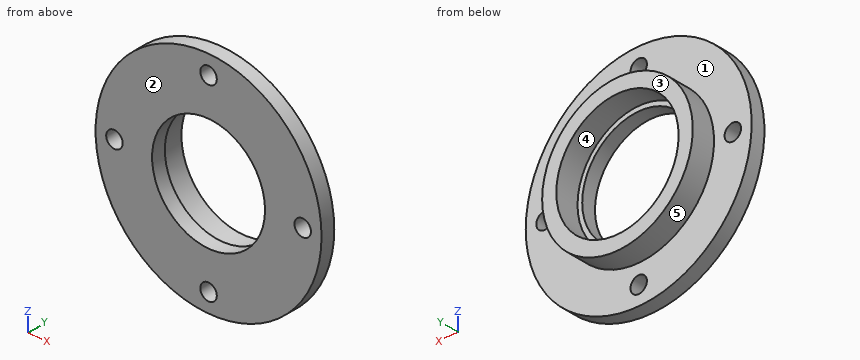
```python
from build123d import *

# Parameters (mm, degrees)
CUT_EXTRUDE_1_DEPTH      = 35.307433597
CUT_EXTRUDE_1_DEPTH_BACK = 35.307433597
SKETCH_2_R               = 1.75


with BuildPart() as part:
    # 草图1 → 旋转1 (revolve)
    with BuildSketch(Plane.XY, mode=Mode.PRIVATE) as revolve_1_sk:
        Polygon((-12, 0), (-24, 0), (-24, 3), (-16, 3), (-16, 8), (-13, 8), (-13, 3), (-12, 3), align=None)
    revolve(revolve_1_sk.sketch.rotate(Axis((0, -271.309816207, 0), (0, 1, 0)), 180), axis=Axis((0, -271.309816207, 0), (0, 1, 0)))

    # 草图2 → 切除-拉伸1 (cut, two sides: drawn at the far end of the back side and taken through both)
    with BuildSketch(Plane(origin=(0, 3, 0), x_dir=(1, 0, 0), z_dir=(0, 1, 0)).offset(-CUT_EXTRUDE_1_DEPTH_BACK)):
        with Locations(Location((0, 20, 0), (0, 0, 180))):
            Circle(SKETCH_2_R)
        with Locations(Location((20, 0, 0), (0, 0, 180))):
            Circle(SKETCH_2_R)
        with Locations(Location((0, -20, 0), (0, 0, 180))):
            Circle(SKETCH_2_R)
        with Locations(Location((-20, 0, 0), (0, 0, 180))):
            Circle(SKETCH_2_R)
    extrude(amount=CUT_EXTRUDE_1_DEPTH + CUT_EXTRUDE_1_DEPTH_BACK, mode=Mode.SUBTRACT)


solid = part.part
```
Geometry check sheet. Reference: the model listing, model coordinates, mm. Face numbers are marked on the shaded views. A direction names the side the tool comes from. Round coordinates to 2 decimals unless told otherwise and drop trailing zeros. Loops run counter-clockwise (first coordinate to the right, second up) from the corner with the lowest first, then second, coordinate; pieces in that order, holes last. Notation, with made-up numbers: M -11,48.25 L 24,48.25 A20 ccw 24,55.25 Z; hole C 3,37.25 d4. An arc over 180 degrees is marked long. Return JSON: item names as keys, results as strings. Group by question number.
(1) Set-up check for the marked faces 1 and 2: record each of +Z, -Z, +X, -X, +Y, -Y from which the full face is reachable in a straight line by a thin tool's end or side.
(2) Section check A-A, the plane z = 0. Enter the section's corners in (x, y).
(3) Section check D-D, the plane x = -20. Enter the section's corners in (y, z), and give its area (3 significant figures).
(4) Section check C-C, the plane z = 20. Enter the section's corners in (x, y), and give its area (3 significant figures).
(5) Mould release check, pull along X, two halves, no side actions. Record for the marked faces 3, 4 and 5: pulls with the +X half, pulls with the -X half, needs draft (parallel to the pull), parting line crosses it, or undercut.
(6) Go/stop test with flat-tipped pins: pin 1 (3 mm diameter, centred on x = -5.5, y = 7, fed in from -Z); pin 2 (4.5 mm diameter, centred on x = 0, z = 20, fed in from -Y); pin 3 (5.5 mm diameter, centred on x = 0, z = -20, fed in from +Y); pin 4 (3 mm diameter, centred on x = -10, y = 4, fed in from -Z). Record where each tip stops, or that it passes through.
(7) Scan lines: line 1 along Z through (x, y) = (0, 2.25); line 2 along Z through (x, y) = (0, 6.8); line 3 along X through (y, z) = (1, 20.5). Record each from-to range of solid material in increasing order. Write a range as [from, to].
(8) Section check B-B, the plane x = 0. Enter the section's corners in (y, z), and give its area (3 significant figures).
Data:
{
 "1": {"face 1": "+Y", "face 2": "+Z, -Z, +X, -X, -Y"},
 "2": {"outline": "M -24,0 L -21.75,0 L -21.75,3 L -24,3 Z; M -18.25,0 L -12,0 L -12,3 L -13,3 L -13,8 L -16,8 L -16,3 L -18.25,3 Z; M 12,0 L 18.25,0 L 18.25,3 L 16,3 L 16,8 L 13,8 L 13,3 L 12,3 Z; M 21.75,0 L 24,0 L 24,3 L 21.75,3 Z"},
 "3": {"outline": "M 0,-13.27 L 3,-13.27 L 3,-1.75 L 0,-1.75 Z; M 0,1.75 L 3,1.75 L 3,13.27 L 0,13.27 Z", "area": "69.1 mm²"},
 "4": {"outline": "M -13.27,0 L -1.75,0 L -1.75,3 L -13.27,3 Z; M 1.75,0 L 13.27,0 L 13.27,3 L 1.75,3 Z", "area": "69.1 mm²"},
 "5": {"face 3": "needs draft", "face 4": "undercut", "face 5": "parting line crosses it"},
 "6": {"pin 1": "z = -15.49", "pin 2": "y = 0", "pin 3": "y = 3", "pin 4": "z = -22.3"},
 "7": {"line 1": "[-24, -21.75], [-18.25, -12], [12, 18.25], [21.75, 24]", "line 2": "[-16, -13], [13, 16]", "line 3": "[-12.48, -1.68], [1.68, 12.48]"},
 "8": {"outline": "M 0,-24 L 3,-24 L 3,-21.75 L 0,-21.75 Z; M 0,-18.25 L 3,-18.25 L 3,-16 L 8,-16 L 8,-13 L 3,-13 L 3,-12 L 0,-12 Z; M 0,12 L 3,12 L 3,13 L 8,13 L 8,16 L 3,16 L 3,18.25 L 0,18.25 Z; M 0,21.75 L 3,21.75 L 3,24 L 0,24 Z", "area": "81.0 mm²"}
}
